from build123d import *

# Parameters (mm, degrees)
ESBO_O1_R                = 1.6
RESSALTO_EXTRUS_O1_DEPTH = 3
FILETE1_R                = 7.5


with BuildPart() as part:
    # Esboço1 → Ressalto-extrusão1 (new body)
    with BuildSketch(Plane.XY):
        Polygon((-8, 14.5), (-8, -14.5), (-5, -14.5), (-5, -17.5), (-8, -17.5), (-8, -31), (8, -31), (8, -17.5), (5, -17.5), (5, -14.5), (8, -14.5), (8, -5), (11, -5), (11, 5), (8, 5), (8, 14.5), (5, 14.5), (5, 17.5), (8, 17.5), (8, 31), (-8, 31), (-8, 17.5), (-5, 17.5), (-5, 14.5), align=None)
        with Locations((0, -25)):
            Circle(ESBO_O1_R, mode=Mode.SUBTRACT)
        with Locations((0, 25)):
            Circle(ESBO_O1_R, mode=Mode.SUBTRACT)
    extrude(amount=RESSALTO_EXTRUS_O1_DEPTH)

    # Filete1
    filete1_edges = [part.edges().sort_by_distance(p)[0] for p in [
        (-8, 31, 1.5),
        (8, 31, 1.5),
        (8, -31, 1.5),
        (-8, -31, 1.5),
    ]]
    fillet(filete1_edges, radius=FILETE1_R)


solid = part.part
Here's how the part is built. I have some questions about the finished solid (model axes, mm). A direction names the side the tool comes from. Coordinates: 2 decimals unless noted, no trailing zeros. Loops run counter-clockwise (first coordinate to the right, second up) from the corner with the lowest first, then second, coordinate; pieces in that order, holes last.
1. For faces 1 (the flat face through (6, 17.5, 1)), 2 (the flat face through (0, 31, 1)), 3 (the flat face through (8, 10, 1)), 4 (the flat face through (-7, -14.5, 1)), which set-ups out of +Z, -Z, +X, -X, +Y, -Y let a thin tool reach every point of the face, with its end or its side?
2. Imagine slicing it at D-D, the plane x = 4. Please give me the cut outline in (y, z), and give its area (3 significant figures).
3. I need wall thicknesses on L1, parallel to Y at x = 0, z = 0.7; L2, parallel to Y at x = 1, z = 1.8; L3, parallel to X at y = 5.5, z = 0.45. Which ranges of each line are inside material? Lowest first, please.
4. Imagine slicing it at A-A, the plane z = 2.1. Count the separate pieces of the cut face and the enclosed holes in it, and give its area (3 significant figures).
5. Imagine slicing it at C-C, the plane x = -6. Please give me the cut outline in (y, z).
6. Imagine slicing it at B-B, the plane y = -25. Please give me the cut outline in (x, z), and give its area (3 significant figures).
7. For P1, Ø4, axis at x = 0, y = -25, coming from the +Z side; P2, Ø1.5, axis at x = 9, z = 1, coming from the -Y side; P3, Ø1.5, axis at x = -6.5, z = 1, coming from the -Y side; P4, Ø0.9, axis at x = 7, z = 1, coming from the -Y side, each with a flat end and sliding along its axis, tell me the tip position at first contact or that it passes through.
8. If we mould it in two halves opening along X, with no side actions, what happens to faces 5 (the flat face through (9, -5, 1)), 6 (the flat face through (-5, -16, 1)), 7 (the flat face through (8, -10, 1)), 8 (the cylindrical face through (-1.27, 24.03, 1.48))? For each: pulls with the +X half, pulls with the -X half, needs draft (parallel to the pull), parting line crosses it, or undercut.
Taken from the geometry:
1. face 1: +Z, -Z, +X
1. face 2: +Z, -Z, +X, -X, +Y
1. face 3: +Z, -Z, +X, +Y
1. face 4: +Z, -Z, -X
2. outline: (-30.13, 0) - (30.13, 0) - (30.13, 3) - (-30.13, 3) - close
2. area: 181 mm2
3. L1: y = -31 to -26.6, -23.4 to 23.4, 26.6 to 31
3. L2: y = -30.98 to -26.25, -23.75 to 23.75, 26.25 to 30.98
3. L3: x = -8 to 8
4. separate pieces: 1
4. enclosed holes: 2
4. area: 922 mm2
5. outline: (-28.6, 0) - (-17.5, 0) - (-17.5, 3) - (-28.6, 3) - close; (-14.5, 0) - (14.5, 0) - (14.5, 3) - (-14.5, 3) - close; (17.5, 0) - (28.6, 0) - (28.6, 3) - (17.5, 3) - close
6. outline: (-7.85, 0) - (-1.6, 0) - (-1.6, 3) - (-7.85, 3) - close; (1.6, 0) - (7.85, 0) - (7.85, 3) - (1.6, 3) - close
6. area: 37.5 mm2
7. P1: stops at z = 3
7. P2: stops at y = -5
7. P3: stops at y = -28.86
7. P4: stops at y = -27.93
8. face 5: needs draft
8. face 6: pulls with the -X half
8. face 7: pulls with the +X half
8. face 8: undercut
